Source: CAD feature listing. Evaluate the final solid. Frame: model axes, mm. Face numbers are marked on the shaded views. A direction names the side the tool comes from. Round coordinates to 2 decimals unless told otherwise and drop trailing zeros. Write each loop counter-clockwise with the first axis right and the second up, starting at its lowest first coordinate (ties: lowest second). Pieces come first, ordered by that corner, then holes. Notation, with made-up numbers: M 2.25,17.25 L 7.25,17.25 A16 ccw 7.25,48.25 Z; hole C 10.5,-3.5 d3. An arc over 180 degrees is marked long. Answer in a Markdown table with one row per item.
from build123d import *

# Parameters (mm, degrees)
F0_W     = 1300
F0_H     = 930
F1_DEPTH = 900
F2_T     = -5
F3_W     = 200
F3_H     = 250
F4_DEPTH = 25
F5_W     = 300
F5_H     = 250
F6_DEPTH = 25


with BuildPart() as f1:
    # F0 (on Front) → F1 (new body)
    with BuildSketch(Plane.XZ):
        with Locations((-607.050044, 412.407453)):
            Rectangle(F0_W, F0_H)
    extrude(amount=F1_DEPTH)

    # F2
    f2_openings = [f1.faces().sort_by_distance(p)[0] for p in [
        (-607.050044, -450, -52.592547),
    ]]
    offset(amount=F2_T, openings=f2_openings)

    # F3 (on face) → F4 (cut)
    with BuildSketch(Plane.XZ.offset(900)):
        with Locations((-957.050044, 372.407453)):
            Rectangle(F3_W, F3_H)
    extrude(amount=-F4_DEPTH, mode=Mode.SUBTRACT)

    # F5 (on face) → F6 (cut)
    with BuildSketch(Plane.XY.offset(877.407453)):
        with Locations((-557.050044, -625)):
            Rectangle(F5_W, F5_H)
    extrude(amount=-F6_DEPTH, mode=Mode.SUBTRACT)


solid = f1.part
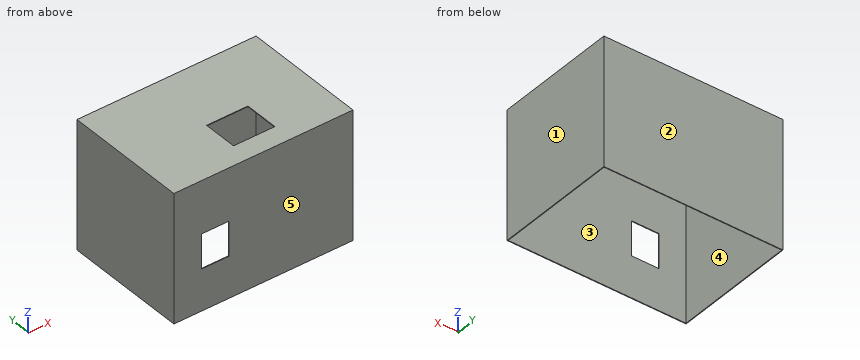
Q1. Pull-direction query (X, two-part tool) for the marked faces 1, 2 and 3; classes: pulls with the +X half, pulls with the -X half, needs draft (parallel to the pull), parting line crosses it, or undercut.
Solutions:
| item | result |
|---|---|
| face 1 | pulls with the +X half |
| face 2 | needs draft |
| face 3 | undercut |
Q2. Section C-C (y = -184). Return loops of the section in (x, z), and give its area (4 significant figures).
Solutions:
| item | result |
|---|---|
| outline | M -1257.05,-52.59 L -1252.05,-52.59 L -1252.05,872.41 L 37.95,872.41 L 37.95,-52.59 L 42.95,-52.59 L 42.95,877.41 L -1257.05,877.41 Z |
| area | 15,750 mm2 |
Q3. Section A-A (x = -1003). Return loops of the section in (y, z), and give its area (3 significant figures).
Solutions:
| item | result |
|---|---|
| outline | M -900,-52.59 L -895,-52.59 L -895,247.41 L -900,247.41 Z; M -900,497.41 L -895,497.41 L -895,872.41 L -5,872.41 L -5,-52.59 L 0,-52.59 L 0,877.41 L -900,877.41 Z |
| area | 12,500 mm2 |
Q4. Contact query for flat-ended pins moving along their axis: pin 1 Ø5 at (x, z) = (-982, 301.5) entering from -Y; pin 2 Ø6 at (x, y) = (-179, -328) entering from -Z. Output: stop coordinate, or through.
Solutions:
| item | result |
|---|---|
| pin 1 | stops at y = -5 |
| pin 2 | stops at z = 872.41 |
Q5. Section D-D (z = 345). Return loops of the section in (x, y), and give its area (3 significant figures).
Solutions:
| item | result |
|---|---|
| outline | M -1257.05,-900 L -1057.05,-900 L -1057.05,-895 L -1252.05,-895 L -1252.05,-5 L 37.95,-5 L 37.95,-895 L -857.05,-895 L -857.05,-900 L 42.95,-900 L 42.95,0 L -1257.05,0 Z |
| area | 20,900 mm2 |
Q6. Section B-B (z = 75). Return loops of the section in (x, y), and give its area (3 significant figures).
Solutions:
| item | result |
|---|---|
| outline | M -1257.05,-900 L 42.95,-900 L 42.95,0 L -1257.05,0 Z; hole M -1252.05,-895 L 37.95,-895 L 37.95,-5 L -1252.05,-5 Z |
| area | 21,900 mm2 |
Q7. Material intervals for probe 1 along Y at (x, z) = (-801.5, 361.5); probe 2 along X at (y, z) = (-784.5, 46); probe 3 along Z at (x, y) = (-163.5, -430.5), sorted ascending.
Solutions:
| item | result |
|---|---|
| probe 1 | y = -900 to -895, -5 to 0 |
| probe 2 | x = -1257.05 to -1252.05, 37.95 to 42.95 |
| probe 3 | z = 872.41 to 877.41 |
Q8. Access query for the marked faces 4 and 5. Directions: +Z, -Z, +X, -X, +Y, -Y. A direction counts if a zero-diameter tool reaches every point of the face in a straight line with its end or side. Return the directions, or none.
Solutions:
| item | result |
|---|---|
| face 4 | -Z |
| face 5 | +Z, -Z, +X, -X, -Y |
